The drawing under review shows one solid part. Ordinate dimensions are in mm from its lowest x, y, z. Give positions to 0.01 mm unless a question says otherwise; leave off trailing zeros. Write each loop counter-clockwise with the first axis right and the second up, starting at its lowest first coordinate (ties: lowest second). Pieces come first, ordered by that corner, then holes. Notation, with made-up numbers: (85, 84.25) -> (93, 84.25) arc R8 ccw to (93, 93.25) -> close; hole circle Ø9 at (35.25, -1). An arc over 180 degrees is marked (long way). Write item = value, one per line.
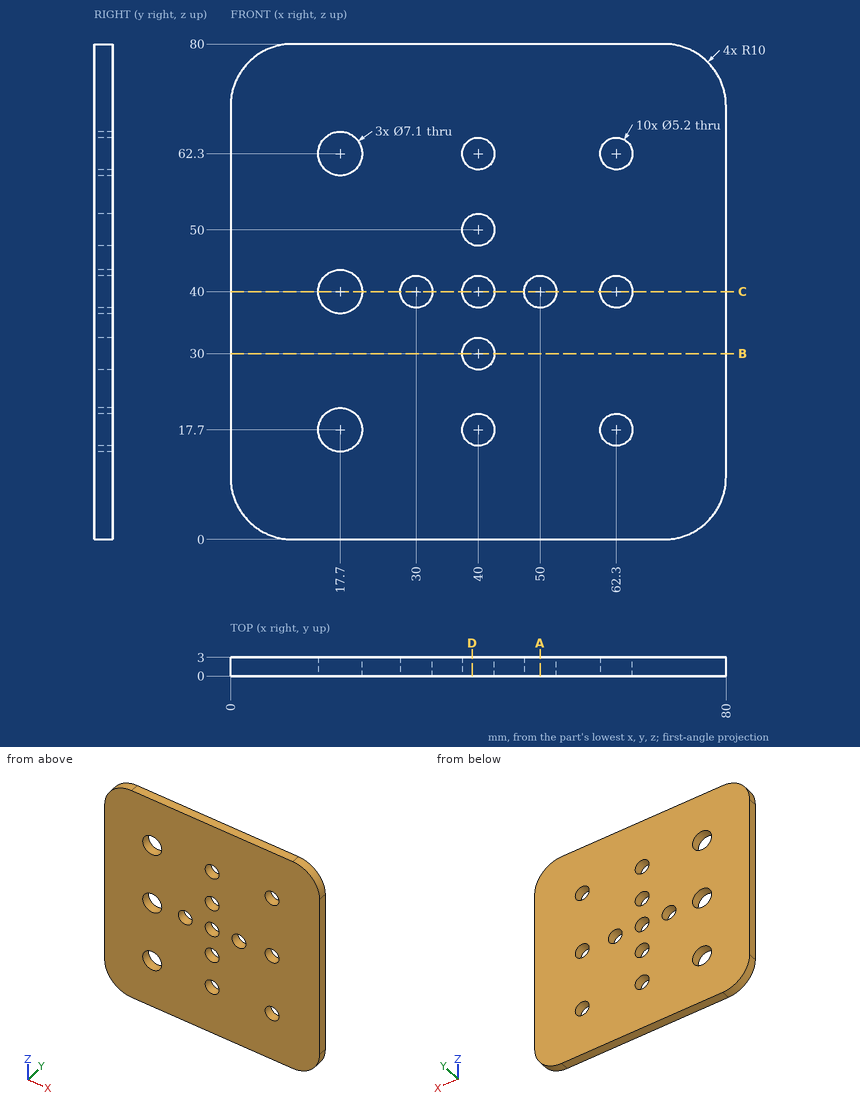
(1) Take a section at A-A (x = 50). Write out the cut boundary in (y, z), plus the area to 3 significant figures.
Answers below:
outline = (0, 0) -> (3, 0) -> (3, 37.4) -> (0, 37.4) -> close; (0, 42.6) -> (3, 42.6) -> (3, 80) -> (0, 80) -> close
area = 224 mm^2
(2) Take a section at C-C (z = 40). Write out the cut boundary in (x, y).
Answers below:
outline = (0, 0) -> (14.15, 0) -> (14.15, 3) -> (0, 3) -> close; (21.25, 0) -> (27.4, 0) -> (27.4, 3) -> (21.25, 3) -> close; (32.6, 0) -> (37.4, 0) -> (37.4, 3) -> (32.6, 3) -> close; (42.6, 0) -> (47.4, 0) -> (47.4, 3) -> (42.6, 3) -> close; (52.6, 0) -> (59.7, 0) -> (59.7, 3) -> (52.6, 3) -> close; (64.9, 0) -> (80, 0) -> (80, 3) -> (64.9, 3) -> close
(3) Take a section at B-B (z = 30). Write out the cut boundary in (x, y).
Answers below:
outline = (0, 0) -> (37.4, 0) -> (37.4, 3) -> (0, 3) -> close; (42.6, 0) -> (80, 0) -> (80, 3) -> (42.6, 3) -> close
(4) To check wall thickness, follow probe 1 along Z at (x, y) = (40, 1.6); probe 2 along Z at (x, y) = (17.7, 1.9); probe 3 along X at (y, z) = (1.1, 62.3). State the ranges of each line that lie inside material, in increasing order.
Answers below:
probe_1 = 0 to 15.1, 20.3 to 27.4, 32.6 to 37.4, 42.6 to 47.4, 52.6 to 59.7, 64.9 to 80
probe_2 = 0 to 14.15, 21.25 to 36.45, 43.55 to 58.75, 65.85 to 80
probe_3 = 0 to 14.15, 21.25 to 37.4, 42.6 to 59.7, 64.9 to 80
(5) Take a section at D-D (x = 39). Write out the cut boundary in (y, z), plus the area to 3 significant figures.
Answers below:
outline = (0, 0) -> (3, 0) -> (3, 15.3) -> (0, 15.3) -> close; (0, 20.1) -> (3, 20.1) -> (3, 27.6) -> (0, 27.6) -> close; (0, 32.4) -> (3, 32.4) -> (3, 37.6) -> (0, 37.6) -> close; (0, 42.4) -> (3, 42.4) -> (3, 47.6) -> (0, 47.6) -> close; (0, 52.4) -> (3, 52.4) -> (3, 59.9) -> (0, 59.9) -> close; (0, 64.7) -> (3, 64.7) -> (3, 80) -> (0, 80) -> close
area = 168 mm^2
